Check sheet for the modelled part. Datum: model origin and axes. Units: mm. Face numbers are marked on the shaded views. Give positions to 0.01 mm unless a question says otherwise; leave off trailing zeros. Loops run counter-clockwise (first coordinate to the right, second up) from the corner with the lowest first, then second, coordinate; pieces in that order, holes last. Notation, with made-up numbers: (32.25, 3.25) - (43.25, 3.25) arc R20 ccw to (43.25, 32.25) - close; hole circle Ø10 at (8.5, 61.25). An arc over 180 degrees is marked (long way). Answer in a Markdown table with one row per item. Add a question column.
(1) Draft check along Z on the marked faces 1, 2, 3 and 4. Enter one of: released by +Z, released by -Z, zero draft, split by the parting line, or undercut.
(2) Sectioned sample at B-B on z = -7. Enter the section's corners in (x, y), then the cut area to 3 significant figures.
(3) Sectioned sample at A-A on x = 0. Enter the section's corners in (y, z), then the cut area to 3 significant figures.
(4) Go/stop test with flat-tipped pins: P1, Ø6, axis at x = 0, z = -14, coming from the +Y side; P2, Ø2, axis at x = -11, z = 7, coming from the +Y side; P3, Ø2, axis at x = 12.12, z = 7, coming from the +Y side. Record where each tip stops, or that it passes through.
(5) Sectioned sample at D-D on x = -12.7. Enter the section's corners in (y, z), then the cut area to 3 significant figures.
(6) Sectioned sample at C-C on z = 12.7. Enter the section's corners in (x, y).
(7) Thickness scan on L1, parallel to X at y = 2.4, z = 0; L2, parallel to X at y = 1.6, z = 7; L3, parallel to X at y = 2.5, z = -12.7. Record the ranges inside material, lowest first.
from build123d import *

# Parameters (mm, degrees)
SKETCH1_W                      = 40
SKETCH1_H                      = 40
BOSS_EXTRUDE1_DEPTH            = 5.5
CUT_EXTRUDE1_REACH             = 30.814
SKETCH2_R                      = 10.5
M3X0_5_TAPPED_HOLE1_D          = 2.5
M3X0_5_TAPPED_HOLE1_DEPTH      = 15.24
M3X0_5_TAPPED_HOLE1_TIP        = 0.751075774
CBORE_FOR_M3_SBHCS1_AT_2_COUNT = 2
CBORE_FOR_M3_SBHCS1_AT_2_PITCH = 7.246933263
CIRPATTERN1_COUNT              = 3


with BuildPart() as part:
    # Sketch1 → Boss-Extrude1 (new body)
    with BuildSketch(Plane(origin=(0, 0, 0), x_dir=(1, 0, 0), z_dir=(0, 1, 0))):
        Rectangle(SKETCH1_W, SKETCH1_H)
    extrude(amount=BOSS_EXTRUDE1_DEPTH)

    # Sketch2 → Cut-Extrude1 (cut, up to next)
    with BuildSketch(Plane(origin=(0, 5.5, 0), x_dir=(1, 0, 0), z_dir=(0, 1, 0)), mode=Mode.PRIVATE) as cut_extrude1_sk1:
        with Locations(Location((0, 0, 0), (0, 0, 270))):
            Circle(SKETCH2_R)
    cut_extrude1_tool1 = extrude(cut_extrude1_sk1.sketch, amount=-CUT_EXTRUDE1_REACH, mode=Mode.PRIVATE) & part.part
    add(cut_extrude1_tool1.solids().sort_by_distance((0, 5.5, 0))[0], mode=Mode.SUBTRACT)

    # M3x0.5 Tapped Hole1
    with Locations(Plane(origin=(0, 5.5, 0), x_dir=(1, 0, 0), z_dir=(0, 1, 0))):
        with Locations((-12.7, -12.7), (-12.7, 12.7), (12.7, 12.7), (12.7, -12.7)):
            Hole(M3X0_5_TAPPED_HOLE1_D / 2, depth=M3X0_5_TAPPED_HOLE1_DEPTH)
            with Locations((0, 0, -(M3X0_5_TAPPED_HOLE1_DEPTH + M3X0_5_TAPPED_HOLE1_TIP / 2))):  # 118° drill point
                Cone(0, M3X0_5_TAPPED_HOLE1_D / 2, M3X0_5_TAPPED_HOLE1_TIP, mode=Mode.SUBTRACT)

    # Sketch10 → CBORE for M3 SBHCS1 (revolve, cut)
    with BuildSketch(Plane(origin=(-12.124355653, 5.5, 7), x_dir=(0, 0, 1), z_dir=(1, 0, 0))):
        Polygon((0, 0), (0, 16.261463052), (1.7, 15.24), (1.7, 1.65), (3.35, 1.65), (3.35, 0), align=None)
    cbore_for_m3_sbhcs1 = revolve(axis=Axis((-12.124355653, 11.85, 7), (0, -1, 0)), mode=Mode.SUBTRACT)

    # CBORE for M3 SBHCS1 at 2: CBORE for M3 SBHCS1 ×2
    with Locations(*[Vector(0.7071067811865501, 0, 0.7071067811865449) * (i * CBORE_FOR_M3_SBHCS1_AT_2_PITCH) for i in range(1, CBORE_FOR_M3_SBHCS1_AT_2_COUNT)]):
        add(cbore_for_m3_sbhcs1, mode=Mode.SUBTRACT)

    # CirPattern1: CBORE for M3 SBHCS1 ×3 about axis
    cirpattern1_axis = Axis((0, 0, 0), (0, 1, 0))
    for i in range(1, CIRPATTERN1_COUNT):
        add(cbore_for_m3_sbhcs1.rotate(cirpattern1_axis, i * 360 / CIRPATTERN1_COUNT), mode=Mode.SUBTRACT)

    # CirPattern1 copy 1 sketch → CirPattern1 copy 1 (revolve, cut)
    with BuildSketch(Plane(origin=(14, 5.5, 0), x_dir=(0.8660254037844387, 0, -0.4999999999999998), z_dir=(-0.4999999999999998, 0, -0.8660254037844387))):
        Polygon((0, 0), (0, 16.261463052), (1.7, 15.24), (1.7, 1.65), (3.35, 1.65), (3.35, 0), align=None)
    revolve(axis=Axis((14, 11.85, 0), (0, -1, 0)), mode=Mode.SUBTRACT)

    # CirPattern1 copy 2 sketch → CirPattern1 copy 2 (revolve, cut)
    with BuildSketch(Plane(origin=(-7, 5.5, -12.124355653), x_dir=(-0.8660254037844384, 0, -0.5000000000000004), z_dir=(-0.5000000000000004, 0, 0.8660254037844384))):
        Polygon((0, 0), (0, 16.261463052), (1.7, 15.24), (1.7, 1.65), (3.35, 1.65), (3.35, 0), align=None)
    revolve(axis=Axis((-7, 11.85, -12.124355653), (0, -1, 0)), mode=Mode.SUBTRACT)


solid = part.part
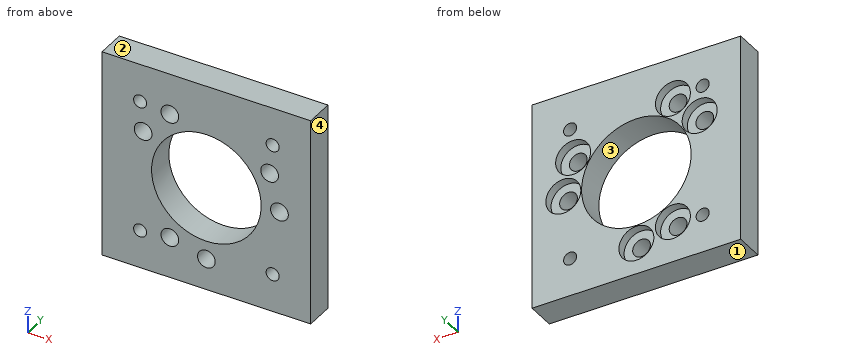
Reply:
| question | item | result |
|---|---|---|
| 1 | face 1 | released by -Z |
| 1 | face 2 | released by +Z |
| 1 | face 3 | undercut |
| 1 | face 4 | zero draft |
| 2 | outline | (-20, 0) - (-7.83, 0) - (-7.83, 5.5) - (-20, 5.5) - close; (7.83, 0) - (20, 0) - (20, 5.5) - (7.83, 5.5) - close |
| 2 | area | 134 mm^2 |
| 3 | outline | (0, -20) - (5.5, -20) - (5.5, -17.35) - (3.85, -17.35) - (3.85, -15.7) - (0, -15.7) - close; (0, -12.3) - (3.85, -12.3) - (3.85, -10.65) - (5.5, -10.65) - (5.5, -10.5) - (0, -10.5) - close; (0, 10.5) - (5.5, 10.5) - (5.5, 20) - (0, 20) - close |
| 3 | area | 80.4 mm^2 |
| 4 | P1 | y = 3.85 |
| 4 | P2 | y = 3.85 |
| 4 | P3 | through |
| 5 | outline | (0, -20) - (5.5, -20) - (5.5, -13.95) - (0, -13.95) - close; (0, -11.45) - (5.5, -11.45) - (5.5, 3.7) - (3.85, 3.7) - (3.85, 5.4) - (0, 5.4) - close; (0, 8.6) - (3.85, 8.6) - (3.85, 10.3) - (5.5, 10.3) - (5.5, 11.45) - (0, 11.45) - close; (0, 13.95) - (5.5, 13.95) - (5.5, 20) - (0, 20) - close |
| 5 | area | 169 mm^2 |
| 6 | outline | (-20, 0) - (-13.95, 0) - (-13.95, 5.5) - (-20, 5.5) - close; (-11.45, 0) - (-8.6, 0) - (-8.6, 3.85) - (-10.3, 3.85) - (-10.3, 5.5) - (-11.45, 5.5) - close; (-5.4, 0) - (11.45, 0) - (11.45, 5.5) - (-3.7, 5.5) - (-3.7, 3.85) - (-5.4, 3.85) - close; (13.95, 0) - (20, 0) - (20, 5.5) - (13.95, 5.5) - close |
| 7 | L1 | -20 to -10.5, 10.5 to 12.3, 15.7 to 20 |
| 7 | L2 | -20 to -13.82, -10.42 to -7.83, 7.83 to 10.42, 13.82 to 20 |
| 7 | L3 | -20 to -13.95, -11.45 to -8.6, -5.4 to -1.1, 1.1 to 11.45, 13.95 to 20 |
